Source: CAD feature listing. Evaluate the final solid. Frame: model axes, mm. A direction names the side the tool comes from. Round coordinates to 2 decimals unless told otherwise and drop trailing zeros. Loops run counter-clockwise (first coordinate to the right, second up) from the corner with the lowest first, then second, coordinate; pieces in that order, holes last. Notation, with made-up numbers: (30, 8) -> (46, 8) arc R18 ccw to (46, 40) -> close; hole circle Ø9 at (20, 12). An arc over 180 degrees is marked (long way). Put each result on its own line as item: value. Start each with the question number.
1. Draft query along Y for faces 1 (the flat face through (-4, 755, 34)), 2 (the flat face through (-66, 0, 3)), 3 (the cylindrical face through (-160.254, 1335.66, 1.972)). Return one class per face: pulls with the +Y half, pulls with the -Y half, needs draft (parallel to the pull), parting line crosses it, or undercut.
2. Contact query for flat-ended pins moving along their axis: pin 1 (5 mm diameter, centred on x = -154.5, y = 753.5, fed in from +Z); pin 2 (2 mm diameter, centred on y = 1097, z = 3, fed in from -X); pin 3 (8 mm diameter, centred on y = 1234.5, z = 22.5, fed in from +X). Output: stop coordinate, or through.
3. Cut plane A-A (x = -123.5). Return the cut outline in (y, z).
4. Set-up query: faces 4 (the flat face through (0, 755, 34)), 5 (the flat face through (-100, 755, 4)). Return all of +Z, -Z, +X, -X, +Y, -Y with unobstructed straight access to the full face (end or side cutting, diameter ignored); none if empty.
5. Cut plane C-C (z = 23.5). Return the cut outline in (x, y).
6. Cut plane D-D (y = 568.5). Return the cut outline in (x, z).
7. Material intervals for L1, parallel to Z at x = -28, y = 277.5; L2, parallel to X at y = 1377, z = 51; L3, parallel to X at y = 280, z = 6.5, sorted ascending.
8. Cut plane B-B (y = 1335). Return the cut outline in (x, z), then the cut area to 3 significant figures.
Autodesk Inventor part; units mm, degrees
ref_plane "YZ Plane" through (0, 0, 0) normal (1, 0, 0) x (0, 1, 0)
ref_plane "XZ Plane" through (0, 0, 0) normal (0, 1, 0) x (-1, 0, 0)
ref_plane "XY Plane" through (0, 0, 0) normal (0, 0, 1) x (1, 0, 0)
sketch "Sketch1" plane through (0, 0, 0) normal (0, 0, 1) x (1, 0, 0)
  line L0 (0, 1490) -> (-190.2469, 1490)
  line L1 (-190.2469, 1490) -> (-190.2469, 0)
  line L2 (-190.2469, 0) -> (0, 0)
  line L3 (0, 0) -> (0, 1490)
  line L4 (-190.2469, 100) -> (-66, 100)
  line L5 (-66, 100) -> (-66, 105)
  line L6 (-66, 105) -> (-190.2469, 105)
  line L7 (-190.2469, 105) -> (-190.2469, 100)
  line L8 (-190.2469, 596.6667) -> (-66, 596.6667)
  line L9 (-66, 596.6667) -> (-66, 601.6667)
  line L10 (-66, 601.6667) -> (-190.2469, 601.6667)
  line L11 (-190.2469, 601.6667) -> (-190.2469, 596.6667)
  line L12 (-190.2469, 1093.3333) -> (-66, 1093.3333)
  line L13 (-66, 1093.3333) -> (-66, 1098.3333)
  line L14 (-66, 1098.3333) -> (-190.2469, 1098.3333)
  line L15 (-190.2469, 1098.3333) -> (-190.2469, 1093.3333)
  circle A0 centre (-190.2469, 1335) radius 30
  point P0 (-190.2469, 1098.3333)
  point P1 (-190.2469, 1093.3333)
  point P2 (-190.2469, 601.6667)
  point P3 (-190.2469, 596.6667)
  point P4 (-190.2469, 1365)
  point P5 (-190.2469, 1305)
  dimension "d0" = 1490
  dimension "d1" = 190.2469
  dimension "d2" = 5
  dimension "d4" = 100
  dimension "d7" = 496.6667
  dimension "d23" = 66
  dimension "d29" = 60
  dimension "d30" = 1335
extrude "Plate1" add sketch "Sketch1" along normal blind 4 contours L3 L2 L1 L4 L5 L6 L8 L9 L10 L12 L13 L14 A0 L0
sketch "Sketch2" plane through (-4, 1490, 0) normal (1, 0, 0) x (0, 1, 0)
  line L0 (-1490, 0) -> (0, 0)
  line L1 (0, 0) -> (0, 60)
  line L2 (0, 60) -> (-1490, 60)
  line L3 (-1490, 60) -> (-1490, 0)
edge flange "Flange1" height 60 angle 90 thickness 4 bend radius 4 thickness toward (1, 0, 0) relief tear relief width 4 relief depth 2 edges at (0, 745, 4) wall of the first edge with corners at (-4, 0, 0) (-4, 1490, 0) (-4, 1490, 60) (-4, 0, 60)
bend "Bend1"
corner "Corner1"
chamfer "Corner Chamfer1" distance 3 angle 45 6 edges at (-190.2469, 100, 2) (-190.2469, 105, 2) (-190.2469, 596.6667, 2) (-190.2469, 601.6667, 2) (-190.2469, 1098.3333, 2) (-190.2469, 1093.3333, 2)
equation "\"d0\" = Стрингер_длина"
equation "\"d1\" = стрингер_глубина_1"
equation "\"d2\" = паз_под_стрингер_толщина"
equation "\"d7\" = Шаг_шпангоутов"
equation "\"d23\" = паз_под_стрингер_глубина - Thickness"
equation "\"d29\" = 2 * радиус_выреза_под_сварку"
equation "\"d12\" = Thickness"
equation "\"d13\" = BendReliefWidth"
equation "\"d14\" = BendReliefDepth"
equation "\"d15\" = MinimumRemnant"
equation "\"d16\" = TransitionRadius"
equation "\"d17\" = ребро_усилителей"
equation "\"d19\" = BendRadius"
equation "\"d20\" = CornerReliefSize"
equation "\"d21\" = GapSize"
equation "\"d22\" = JacobiRadiusSize"
equation "\"BendRadius\" = Thickness"
equation "\"BendReliefWidth\" = Thickness"
equation "\"BendReliefDepth\" = 0.5 * Thickness"
equation "\"CornerReliefSize\" = 4 * Thickness"
equation "\"MinimumRemnant\" = 2 * Thickness"
equation "\"TransitionRadius\" = BendRadius"
equation "\"JacobiRadiusSize\" = BendRadius"
equation "\"GapSize\" = Thickness"
properties part number "GBK 0102 stringer 1" material "Steel"
Solution:
1. face 1: needs draft
1. face 2: pulls with the -Y half
1. face 3: undercut
2. pin 1: stops at z = 4
2. pin 2: stops at x = -66
2. pin 3: stops at x = 0
3. outline: (0, 0) -> (100, 0) -> (100, 4) -> (0, 4) -> close; (105, 0) -> (596.67, 0) -> (596.67, 4) -> (105, 4) -> close; (601.67, 0) -> (1093.33, 0) -> (1093.33, 4) -> (601.67, 4) -> close; (1098.33, 0) -> (1490, 0) -> (1490, 4) -> (1098.33, 4) -> close
4. face 4: +Z, -Z, +X, +Y, -Y
4. face 5: +Z, -X, +Y, -Y
5. outline: (-4, 0) -> (0, 0) -> (0, 1490) -> (-4, 1490) -> close
6. outline: (-190.25, 0) -> (-8, 0) arc R8 ccw to (0, 8) -> (0, 60) -> (-4, 60) -> (-4, 8) arc R4 cw to (-8, 4) -> (-190.25, 4) -> close
7. L1: z = 0 to 4
7. L2: x = -4 to 0
7. L3: x = -4.29 to -0.14
8. outline: (-160.25, 0) -> (-8, 0) arc R8 ccw to (0, 8) -> (0, 60) -> (-4, 60) -> (-4, 8) arc R4 cw to (-8, 4) -> (-160.25, 4) -> close
8. area: 855 mm^2
